```python
from build123d import *

# Parameters (mm, degrees)
BOSS_EXTRUDE1_DEPTH = 5.715
SKETCH4_W           = 3.81
SKETCH4_H           = 55.271796861
CUT_EXTRUDE3_DEPTH  = 72.793515752
SKETCH6_R           = 1.905
CUT_EXTRUDE5_DEPTH  = 73.472702303
SKETCH5_W           = 6.604
SKETCH5_H           = 15.494
CUT_EXTRUDE4_DEPTH  = 52.07
BOSS_EXTRUDE2_DEPTH = 1.905
BOSS_EXTRUDE3_DEPTH = 1.2


with BuildPart() as part:
    # Sketch1 → Boss-Extrude1 (new, symmetric)
    with BuildSketch(Plane(origin=(0, 0, 0), x_dir=(0, 0, -1), z_dir=(1, 0, 0))):
        with BuildLine():
            Line((56.986930037, 27.2309067), (49.395231729, 32.546671083))
            ThreePointArc((49.395231729, 32.546671083), (47.938347581, 33.00602489), (46.481463433, 32.546671083))
            Line((46.481463433, 32.546671083), (36.982659893, 25.89553724))
            ThreePointArc((36.982659893, 25.89553724), (36.033680051, 24.629396088), (36.018345244, 23.047169493))
            Line((36.018345244, 23.047169493), (51.273584689, -25.063981175))
            ThreePointArc((51.273584689, -25.063981175), (52.194518967, -26.3458465), (53.694783485, -26.836259621))
            Line((53.694783485, -26.836259621), (55.908973953, -26.836259621))
            ThreePointArc((55.908973953, -26.836259621), (57.301856909, -26.420283413), (58.238514534, -25.308603771))
            ThreePointArc((58.238514534, -25.308603771), (63.498135482, 0.4866111), (57.843797801, 26.198188029))
            ThreePointArc((57.843797801, 26.198188029), (57.484796778, 26.772157225), (56.986930037, 27.2309067))
        make_face()
    extrude(amount=BOSS_EXTRUDE1_DEPTH, both=True)

    # Sketch4 → Cut-Extrude3 (cut, through all)
    with BuildSketch(Plane.XY):
        with Locations((0, -1.74036119)):
            Rectangle(SKETCH4_W, SKETCH4_H)
    extrude(amount=-CUT_EXTRUDE3_DEPTH, mode=Mode.SUBTRACT)

    # Sketch6 → Cut-Extrude5 (cut, through all)
    with BuildSketch(Plane(origin=(5.715, 0, 0), x_dir=(0, 0, -1), z_dir=(1, 0, 0))):
        with Locations((38.439544041, 23.814891048)):
            Circle(SKETCH6_R)
    extrude(amount=-CUT_EXTRUDE5_DEPTH, mode=Mode.SUBTRACT)

    # Sketch5 → Cut-Extrude4 (cut)
    with BuildSketch(Plane.XY):
        with Locations((0, 13.527891048)):
            Rectangle(SKETCH5_W, SKETCH5_H)
    extrude(amount=-CUT_EXTRUDE4_DEPTH, mode=Mode.SUBTRACT)

    # Sketch7 → Boss-Extrude2 (add)
    with BuildSketch(Plane(origin=(0, 45.047311475, -31.542467071), x_dir=(1, 0, 0), z_dir=(0, 0.8191520442889956, -0.5735764363510407))):
        with BuildLine():
            Line((1.524, 25.981953814), (-1.524, 25.981953814))
            ThreePointArc((-1.524, 25.981953814), (-2.422025612, 26.353928202), (-2.794, 27.251953814))
            Line((-2.794, 27.251953814), (-2.794, 31.061953814))
            Line((-2.794, 31.061953814), (2.794, 31.061953814))
            Line((2.794, 31.061953814), (2.794, 27.251953814))
            ThreePointArc((2.794, 27.251953814), (2.422025612, 26.353928202), (1.524, 25.981953814))
        make_face()
    extrude(amount=BOSS_EXTRUDE2_DEPTH)

    # Sketch9 → Boss-Extrude3 (add)
    with BuildSketch(Plane(origin=(0, 46.607796119, -32.635130182), x_dir=(1, 0, 0), z_dir=(0, 0.8191520442889956, -0.5735764363510407))):
        with BuildLine():
            Line((2.890823379, 31.061953814), (-2.890823379, 31.061953814))
            ThreePointArc((-2.890823379, 31.061953814), (-3.788848991, 30.689979426), (-4.160823379, 29.791953814))
            Line((-4.160823379, 29.791953814), (-4.160823379, 25.346953814))
            ThreePointArc((-4.160823379, 25.346953814), (-3.788848991, 24.448928202), (-2.890823379, 24.076953814))
            Line((-2.890823379, 24.076953814), (2.890823379, 24.076953814))
            ThreePointArc((2.890823379, 24.076953814), (3.788848991, 24.448928202), (4.160823379, 25.346953814))
            Line((4.160823379, 25.346953814), (4.160823379, 29.791953814))
            ThreePointArc((4.160823379, 29.791953814), (3.788848991, 30.689979426), (2.890823379, 31.061953814))
        make_face()
    extrude(amount=BOSS_EXTRUDE3_DEPTH)


solid = part.part
```
Work out the finished part from the listing and answer in its coordinate system (mm). A direction names the side the tool comes from. Coordinates: 2 decimals unless noted, no trailing zeros. Loops run counter-clockwise (first coordinate to the right, second up) from the corner with the lowest first, then second, coordinate; pieces in that order, holes last. Notation, with made-up numbers: (44, 24.5) - (59, 24.5) arc R23 ccw to (59, 36.5) - close; hole circle Ø7 at (77.25, 4.25). An arc over 180 degrees is marked (long way). Use a Markdown table: item, result.
Item 1: For faces 5 (the flat face through (-1.905, -1, -53)), 6 (the cylindrical face through (2.432, 30.695, -53.677)), 7 (the flat face through (3, 14, -52.07)), 8 (the cylindrical face through (-3.8, 33.06, -53.01)), determine the directions among +Z, -Z, +X, -X, +Y, -Y from which every point of the face is accessible in a straight line to the end or side of a thin tool.
Evaluation:
| item | result |
|---|---|
| face 5 | +Z, -Z, -Y |
| face 6 | +X |
| face 7 | +Z |
| face 8 | -X, +Y |
Item 2: Find section C-C, the plane z = -61.5. Determine the outline of the cut face in (x, y) (3 decimals), and give its area (3 significant figures).
Evaluation:
| item | result |
|---|---|
| outline | (-5.715, -15.811) - (-1.905, -15.811) - (-1.905, 15.811) - (-5.715, 15.811) - close; (1.905, -15.811) - (5.715, -15.811) - (5.715, 15.811) - (1.905, 15.811) - close |
| area | 241 mm2 |
Item 3: The mould has two halves that part along Z. Classify faces 1 (the flat face through (-3, 21.275, -44)), 2 (the cylindrical face through (-3.783, -26.432, -57.285)), 3 (the flat face through (0.02, 30.91, -53.36)), 4 (the flat face through (0.08, 30.442, -52.401)): +Z half, -Z half, draft (parallel to the pull), parting line (faces both ways), or undercut.
Evaluation:
| item | result |
|---|---|
| face 1 | draft |
| face 2 | -Z half |
| face 3 | undercut |
| face 4 | undercut |
Item 4: Given pin 1 Ø1.1 at (x, z) = (2.5, -49) entering from +Y; pin 2 Ø2 at (x, y) = (2, -6) entering from +Z; pin 3 Ø3 at (y, z) = (31.5, -56) entering from +X; pin 4 Ø3.5 at (y, z) = (23.81, -38.44) entering from +X, each flat-ended and moving along its own axis, determine where each tip first touches the part or whether it passes through.
Evaluation:
| item | result |
|---|---|
| pin 1 | stops at y = 32.95 |
| pin 2 | stops at z = -44.91 |
| pin 3 | stops at x = 4.16 |
| pin 4 | passes through |
Item 5: Find section B-B, the plane x = 0.25. Determine the outline of the cut face in (y, z).
Evaluation:
| item | result |
|---|---|
| outline | (25.9, -57.98) arc R63.5 ccw to (26.2, -57.84) arc R2.54 ccw to (27.23, -56.99) - (29.77, -58.77) - (33.78, -53.05) - (32.8, -52.36) - (31.71, -53.92) - (30.14, -52.83) - (32.55, -49.4) arc R2.54 ccw to (32.55, -46.48) - (25.9, -36.98) - close |
Item 6: Find section A-A, the plane y = -21.5. Determine the outline of the cut face in (x, z) (1 decimal), and give its area (3 significant figures).
Evaluation:
| item | result |
|---|---|
| outline | (-5.7, -59.7) - (-1.9, -59.7) - (-1.9, -50.1) - (-5.7, -50.1) - close; (1.9, -59.7) - (5.7, -59.7) - (5.7, -50.1) - (1.9, -50.1) - close |
| area | 73.2 mm2 |
Item 7: Find section D-D, the plane y = 22.5. Determine the outline of the cut face in (x, z) (3 decimals), and give its area (3 significant figures).
Evaluation:
| item | result |
|---|---|
| outline | (-5.715, -59.38) - (-1.905, -59.38) - (-1.905, -39.818) - (-5.715, -39.818) - close; (-5.715, -37.061) - (-1.905, -37.061) - (-1.905, -36.192) - (-5.715, -36.192) - close; (1.905, -59.38) - (5.715, -59.38) - (5.715, -39.818) - (1.905, -39.818) - close; (1.905, -37.061) - (5.715, -37.061) - (5.715, -36.192) - (1.905, -36.192) - close |
| area | 156 mm2 |
Item 8: Consider probe 1 along X at (y, z) = (18, -51.75) (3 decimals); probe 2 along X at (y, z) = (-1.5, -46.75) (3 decimals); probe 3 along Y at (x, z) = (2, -37.5). Determine where each line is inside the solid, lowest interval first. Write a range as from..to.
Evaluation:
| item | result |
|---|---|
| probe 1 | x = -5.715..-3.302, 3.302..5.715 |
| probe 2 | x = -5.715..-1.905, 1.905..5.715 |
| probe 3 | y = 21.27..22.16, 25.47..26.26 |
